Check sheet for the modelled part. Datum: model origin and axes. Units: mm. Face numbers are marked on the shaded views. A direction names the side the tool comes from. Give positions to 0.01 mm unless a question says otherwise; leave off trailing zeros. Order: outer loops, then holes, each group sorted by start corner. A loop starts at its lowest first (then second) coordinate and runs counter-clockwise, first axis right, second up. Notation, with made-up numbers: M 18.5,-29.75 L 71.5,-29.75 A22 cw 71.5,9.25 Z; hole C 84,25 d10. An arc over 180 degrees is marked long. Answer in a Markdown table with one row per item. Add a question column.
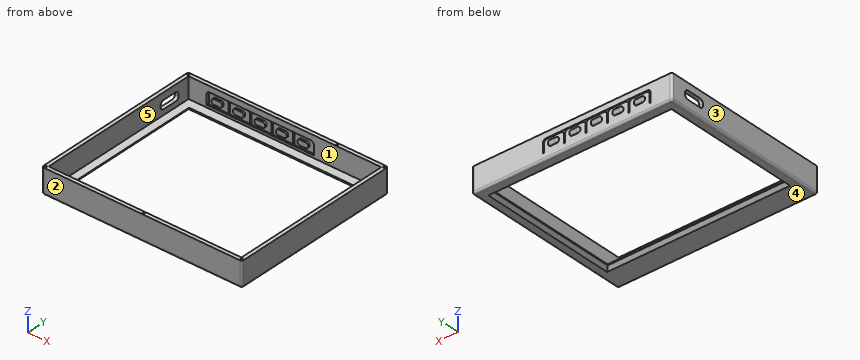
from build123d import *

# Parameters (mm, degrees)
SKETCH009_R      = 0.5
EXTRUDE011_DEPTH = 8
SKETCH010_R      = 0.95
EXTRUDE010_DEPTH = 0.8
SKETCH006_W      = 5
SKETCH006_H      = 2.5
EXTRUDE007_DEPTH = 3
FILLET003_R      = 1
EXTRUDE005_DEPTH = 4
EXTRUDE004_DEPTH = 1
SKETCH003_W      = 62
SKETCH003_H      = 1.7
EXTRUDE003_DEPTH = 4
SKETCH002_W      = 10
SKETCH002_H      = 4
EXTRUDE002_DEPTH = 10
SKETCH_W         = 96
SKETCH_H         = 82
SKETCH_W_2       = 92.5
SKETCH_H_2       = 78.5
EXTRUDE001_DEPTH = 10
FILLET_R         = 1.5
SKETCH001_W      = 96
SKETCH001_H      = 82
SKETCH001_W_2    = 84.8
SKETCH001_H_2    = 63.6
EXTRUDE_DEPTH    = 2
CHAMFER_SIZE     = 1.5
FILLET001_R      = 1
FILLET002_R      = 1.5


with BuildPart() as extrude011:
    # Sketch009 (on Face5 of Fusion002) → Extrude011 (new body)
    with BuildSketch(Plane.XY.offset(12)):
        with Locations((24.37, 40)):
            Circle(SKETCH009_R)
        with Locations((0, -40)):
            Circle(SKETCH009_R)
        with Locations((47, -40)):
            Circle(SKETCH009_R)
        with Locations((-47, -40)):
            Circle(SKETCH009_R)
        with Locations((-47, 40)):
            Circle(SKETCH009_R)
        with Locations((47, 40)):
            Circle(SKETCH009_R)
    extrude(amount=-EXTRUDE011_DEPTH)


with BuildPart() as fusion003:
    # Sketch010 (on Face5 of Fusion002) → Extrude010 (new body)
    with BuildSketch(Plane.XY.offset(12)):
        with Locations((24.37, 40)):
            Circle(SKETCH010_R)
        with Locations((0, -40)):
            Circle(SKETCH010_R)
        with Locations((47, -40)):
            Circle(SKETCH010_R)
        with Locations((-47, -40)):
            Circle(SKETCH010_R)
        with Locations((-47, 40)):
            Circle(SKETCH010_R)
        with Locations((47, 40)):
            Circle(SKETCH010_R)
    extrude(amount=-EXTRUDE010_DEPTH)

    # Fusion003: union Extrude011
    add(extrude011.part)


with BuildPart() as fillet003:
    # Sketch006 (on Face2 of Part__Feature059) → Extrude007 (new body)
    with BuildSketch(Plane(origin=(0, 39, 0), x_dir=(-1, 0, 0), z_dir=(0, 1, 0))):
        with Locations((-8.74, 4.15)):
            Rectangle(SKETCH006_W, SKETCH006_H)
        with Locations((11.9, 4.15)):
            Rectangle(SKETCH006_W, SKETCH006_H)
        with Locations((22.22, 4.15)):
            Rectangle(SKETCH006_W, SKETCH006_H)
        with Locations((32.54, 4.15)):
            Rectangle(SKETCH006_W, SKETCH006_H)
        with Locations((1.58, 4.15)):
            Rectangle(SKETCH006_W, SKETCH006_H)
    extrude(amount=EXTRUDE007_DEPTH)

    # Fillet003
    fillet003_edges = [fillet003.edges().sort_by_distance(p)[0] for p in [
        (-30.04, 40.5, 5.4),
        (-35.04, 40.5, 5.4),
        (-32.54, 42, 5.4),
        (-35.04, 40.5, 2.9),
        (-35.04, 42, 4.15),
        (-30.04, 40.5, 2.9),
        (-32.54, 42, 2.9),
        (-30.04, 42, 4.15),
        (-19.72, 40.5, 5.4),
        (-24.72, 40.5, 5.4),
        (-22.22, 42, 5.4),
        (-24.72, 40.5, 2.9),
        (-24.72, 42, 4.15),
        (-19.72, 40.5, 2.9),
        (-22.22, 42, 2.9),
        (-19.72, 42, 4.15),
        (-9.4, 40.5, 5.4),
        (-14.4, 40.5, 5.4),
        (-11.9, 42, 5.4),
        (-14.4, 40.5, 2.9),
        (-14.4, 42, 4.15),
        (-9.4, 40.5, 2.9),
        (-11.9, 42, 2.9),
        (-9.4, 42, 4.15),
        (11.24, 40.5, 5.4),
        (6.24, 40.5, 5.4),
        (8.74, 42, 5.4),
        (6.24, 40.5, 2.9),
        (6.24, 42, 4.15),
        (11.24, 40.5, 2.9),
        (8.74, 42, 2.9),
        (11.24, 42, 4.15),
        (0.92, 40.5, 5.4),
        (-4.08, 40.5, 5.4),
        (-1.58, 42, 5.4),
        (-4.08, 40.5, 2.9),
        (-4.08, 42, 4.15),
        (0.92, 40.5, 2.9),
        (-1.58, 42, 2.9),
        (0.92, 42, 4.15),
    ]]
    fillet(fillet003_edges, radius=FILLET003_R)


with BuildPart() as extrude005:
    # Sketch005 (on Face2 of Part__Feature059) → Extrude005 (new body)
    with BuildSketch(Plane(origin=(0, 39, 0), x_dir=(-1, 0, 0), z_dir=(0, 1, 0))):
        Polygon((-13.9, 7.2), (37.7, 7.2), (37.7, 1.2), (37.2, 1.2), (37.2, 6.7), (27.63, 6.7), (27.63, 1.2), (27.13, 1.2), (27.13, 6.7), (17.31, 6.7), (17.31, 1.2), (16.81, 1.2), (16.81, 6.7), (6.99, 6.7), (6.99, 1.2), (6.49, 1.2), (6.49, 6.7), (-3.33, 6.7), (-3.33, 1.2), (-3.83, 1.2), (-3.83, 6.7), (-13.4, 6.7), (-13.4, 1.2), (-13.9, 1.2), align=None)
    extrude(amount=EXTRUDE005_DEPTH)


with BuildPart() as extrude004:
    # Sketch004 (on Face2 of Part__Feature059) → Extrude004 (new body)
    with BuildSketch(Plane(origin=(0, 39, 0), x_dir=(-1, 0, 0), z_dir=(0, 1, 0))):
        Polygon((-13.9, 7.2), (37.7, 7.2), (37.7, 1.2), (27.38, 1.2), (17.06, 1.2), (6.74, 1.2), (-3.58, 1.2), (-13.9, 1.2), align=None)
    extrude(amount=EXTRUDE004_DEPTH)


with BuildPart() as extrude003:
    # Sketch003 → Extrude003 (new body)
    with BuildSketch(Plane.XY):
        with Locations((11, -39.15)):
            Rectangle(SKETCH003_W, SKETCH003_H)
    extrude(amount=EXTRUDE003_DEPTH)


with BuildPart() as usb:
    # Sketch002 (on Face4 of Extrude001) → Extrude002 (new body)
    with BuildSketch(Plane(origin=(-48, 0, 0), x_dir=(0, -1, 0), z_dir=(-1, 0, 0))):
        with Locations((-28.62, 4.6)):
            Rectangle(SKETCH002_W, SKETCH002_H)
    extrude(amount=-EXTRUDE002_DEPTH)


with BuildPart() as fillet_body:
    # Sketch → Extrude001 (new body)
    with BuildSketch(Plane.XY):
        Rectangle(SKETCH_W, SKETCH_H)
        Rectangle(SKETCH_W_2, SKETCH_H_2, mode=Mode.SUBTRACT)
    extrude(amount=EXTRUDE001_DEPTH)

    # Cut: cut usb
    add(usb.part, mode=Mode.SUBTRACT)

    # Fillet
    fillet_edges = [fillet_body.edges().sort_by_distance(p)[0] for p in [
        (-47.125, 33.62, 6.6),
        (-47.125, 33.62, 2.6),
        (-47.125, 23.62, 2.6),
        (-47.125, 23.62, 6.6),
    ]]
    fillet(fillet_edges, radius=FILLET_R)


with BuildPart() as font001:
    # Sketch001 (on Face4 of Part__Feature059) → Extrude (new body)
    with BuildSketch(Plane(origin=(0, 0, 0), x_dir=(1, 0, 0), z_dir=(0, 0, -1))):
        Rectangle(SKETCH001_W, SKETCH001_H)
        with Locations((0, -3.2)):
            Rectangle(SKETCH001_W_2, SKETCH001_H_2, mode=Mode.SUBTRACT)
    extrude(amount=EXTRUDE_DEPTH)

    # Chamfer
    chamfer_edges = [font001.edges().sort_by_distance(p)[0] for p in [
        (0, -28.6, -2),
        (42.4, 3.2, -2),
        (0, 35, -2),
        (-42.4, 3.2, -2),
    ]]
    chamfer(chamfer_edges, length=CHAMFER_SIZE)

    # Fusion: union Fillet body
    add(fillet_body.part)

    # Fillet001
    fillet001_edges = [font001.edges().sort_by_distance(p)[0] for p in [
        (0, -41, -2),
        (48, 0, -2),
        (0, 41, -2),
        (-48, 0, -2),
        (-48, -41, -1),
        (48, -41, -1),
        (48, 41, -1),
        (-48, 41, -1),
    ]]
    fillet(fillet001_edges, radius=FILLET001_R)

    # Cut001: cut Extrude003
    add(extrude003.part, mode=Mode.SUBTRACT)

    # Cut002: cut Extrude004
    add(extrude004.part, mode=Mode.SUBTRACT)

    # Cut003: cut Extrude005
    add(extrude005.part, mode=Mode.SUBTRACT)

    # Fillet002
    fillet002_edges = [font001.edges().sort_by_distance(p)[0] for p in [
        (13.4, 40.5, 6.7),
        (3.83, 40.5, 6.7),
        (3.33, 40.5, 6.7),
        (-6.49, 40.5, 6.7),
        (-6.99, 40.5, 6.7),
        (-16.81, 40.5, 6.7),
        (-17.31, 40.5, 6.7),
        (-27.13, 40.5, 6.7),
        (-27.63, 40.5, 6.7),
        (-37.2, 40.5, 6.7),
        (-37.7, 40.5, 7.2),
        (13.9, 40.5, 7.2),
    ]]
    fillet(fillet002_edges, radius=FILLET002_R)

    # Fusion001: union Fillet003
    add(fillet003.part)

    # Cut005: cut Fusion003
    add(fusion003.part, mode=Mode.SUBTRACT)


solid = font001.part
Q1. Thickness scan on probe 1 along X at (y, z) = (-40, 5.65); probe 2 along Y at (x, z) = (24.37, 6); probe 3 along Y at (x, z) = (47, 8.45). Record the ranges inside material, lowest first.
Q2. Draft check along X on the marked faces 1, 2 and 3. Enter one of: pulls with the +X half, pulls with the -X half, needs draft (parallel to the pull), parting line crosses it, or undercut.
Q3. Cross-section at A-A (y = 18). Record the boundary of the cut face in (x, z), and give its area (3 significant figures).
Q4. Tool access check on the marked faces 4 and 5. Record the directions out of +Z, -Z, +X, -X, +Y, -Y that give a thin tool (end or side, any length) a straight path to the whole face; none if there is none.
Q5. Cross-section at C-C (x = 18). Record the boundary of the cut face in (y, z).
Q6. Go/stop test with flat-tipped pins: pin 1 (3 mm diameter, centred on x = 22.5, z = 4.5, fed in from +Y); pin 2 (0.5 mm diameter, centred on y = 40.5, z = 2.5, fed in from -X); pin 3 (0.8 mm diameter, centred on y = 40.5, z = 2.5, fed in from +X) (3 decimals); pin 4 (1.9 mm diameter, centred on x = -47.5, y = 29, fed in from -Z). Record where each tip stops, or that it passes through.
Q7. Cross-section at B-B (y = 27.5). Record the boundary of the cut face in (x, z).
Values follow:
| question | item | result |
|---|---|---|
| 1 | probe 1 | -48 to -47.5, -46.5 to -0.5, 0.5 to 46.5, 47.5 to 48 |
| 1 | probe 2 | -41 to -39.25, 39.25 to 39.5, 40.5 to 41 |
| 1 | probe 3 | -41 to -40.5, -39.5 to 39.5, 40.5 to 41 |
| 2 | face 1 | undercut |
| 2 | face 2 | needs draft |
| 2 | face 3 | pulls with the -X half |
| 3 | outline | M -48,-1 A1 ccw -47,-2 L -43.9,-2 L -42.4,-0.5 L -42.4,0 L -46.25,0 L -46.25,10 L -48,10 Z; M 42.4,-0.5 L 43.9,-2 L 47,-2 A1 ccw 48,-1 L 48,10 L 46.25,10 L 46.25,0 L 42.4,0 Z |
| 3 | area | 54.7 mm² |
| 4 | face 4 | -Z, +X, -X, +Y, -Y |
| 4 | face 5 | +Z |
| 5 | outline | M -41,-1 A1 ccw -40,-2 L -30.1,-2 L -28.6,-0.5 L -28.6,0 L -40,0 L -40,4 L -39.25,4 L -39.25,10 L -41,10 Z; M 35,-0.5 L 36.5,-2 L 40,-2 A1 ccw 41,-1 L 41,10 L 39.25,10 L 39.25,0 L 35,0 Z |
| 6 | pin 1 | y = 41 |
| 6 | pin 2 | x = -47.97 |
| 6 | pin 3 | x = 47.995 |
| 6 | pin 4 | z = -2 |
| 7 | outline | M -48,-1 A1 ccw -47,-2 L -43.9,-2 L -42.4,-0.5 L -42.4,0 L -46.25,0 L -46.25,2.6 L -48,2.6 Z; M -48,6.6 L -46.25,6.6 L -46.25,10 L -48,10 Z; M 42.4,-0.5 L 43.9,-2 L 47,-2 A1 ccw 48,-1 L 48,10 L 46.25,10 L 46.25,0 L 42.4,0 Z |
